from build123d import *

# Parameters (mm, degrees)
F0_W     = 65
F0_H     = 49
F0_R     = 4.5
F1_DEPTH = 1
F0_R_2   = 1.5
F3_DEPTH = 8
F4_R     = 8


with BuildPart() as f1:
    # F0 (on Top) → F1 (new body)
    with BuildSketch(Plane.XY):
        Rectangle(F0_W, F0_H)
        with Locations((-26.5, -18.5)):
            Circle(F0_R, mode=Mode.SUBTRACT)
        with Locations((26.5, -18.5)):
            Circle(F0_R, mode=Mode.SUBTRACT)
        with Locations((-26.5, 18.5)):
            Circle(F0_R, mode=Mode.SUBTRACT)
        with Locations((26.5, 18.5)):
            Circle(F0_R, mode=Mode.SUBTRACT)
    extrude(amount=F1_DEPTH)

    # F0 (on Top) → F3 (join)
    with BuildSketch(Plane.XY):
        with Locations((26.5, 18.5)):
            Circle(F0_R)
        with Locations((26.5, 18.5)):
            Circle(F0_R_2, mode=Mode.SUBTRACT)
        with Locations((-26.5, -18.5)):
            Circle(F0_R)
        with Locations((-26.5, -18.5)):
            Circle(F0_R_2, mode=Mode.SUBTRACT)
        with Locations((-26.5, 18.5)):
            Circle(F0_R)
        with Locations((-26.5, 18.5)):
            Circle(F0_R_2, mode=Mode.SUBTRACT)
        with Locations((26.5, -18.5)):
            Circle(F0_R)
        with Locations((26.5, -18.5)):
            Circle(F0_R_2, mode=Mode.SUBTRACT)
    extrude(amount=F3_DEPTH)

    # F4
    f4_edges = [f1.edges().sort_by_distance(p)[0] for p in [
        (32.5, -24.5, 0.5),
        (32.5, 24.5, 0.5),
        (-32.5, -24.5, 0.5),
        (-32.5, 24.5, 0.5),
    ]]
    fillet(f4_edges, radius=F4_R)


solid = f1.part
Model file for the job. Use its own axes, mm. A direction names the side the tool comes from. Give positions to 0.01 mm unless a question says otherwise; leave off trailing zeros. Write each loop counter-clockwise with the first axis right and the second up, starting at its lowest first coordinate (ties: lowest second). Pieces come first, ordered by that corner, then holes. Notation, with made-up numbers: (-34.75, 40.5) -> (-22.75, 40.5) arc R17 cw to (-22.75, 71.5) -> close; hole circle Ø4 at (79, 60.5). An arc over 180 degrees is marked (long way). Write item = value, one per line.
(1) Slice it at C-C, the plane y = -18.5. Give the cut face in (x, z).
Determined:
outline = (-32.25, 0) -> (-28, 0) -> (-28, 8) -> (-31, 8) -> (-31, 1) -> (-32.25, 1) -> close; (-25, 0) -> (25, 0) -> (25, 8) -> (22, 8) -> (22, 1) -> (-22, 1) -> (-22, 8) -> (-25, 8) -> close; (28, 0) -> (32.25, 0) -> (32.25, 1) -> (31, 1) -> (31, 8) -> (28, 8) -> close
(2) Probe line 1 along Y through (x, z) = (26.5, 5.25); line 2 along Z through (x, y) = (-1, -11); line 3 along X through (y, z) = (-16, 7.5). List the from-to ranges inside material, lowest first.
Determined:
line_1 = -23 to -20, -17 to -14, 14 to 17, 20 to 23
line_2 = 0 to 1
line_3 = -30.24 to -22.76, 22.76 to 30.24
(3) Flat gauge pin, fed straight in: P1, Ø2, axis at x = -2, y = 18, coming from the +Z side. Where does the tip first touch, or does it go through?
Determined:
P1 = 1
(4) Slice it at B-B, the plane x = 26.5. Give the cut face in (y, z), then the cut area to 3 significant figures.
Determined:
outline = (-24.25, 0) -> (-20, 0) -> (-20, 8) -> (-23, 8) -> (-23, 1) -> (-24.25, 1) -> close; (-17, 0) -> (17, 0) -> (17, 8) -> (14, 8) -> (14, 1) -> (-14, 1) -> (-14, 8) -> (-17, 8) -> close; (20, 0) -> (24.25, 0) -> (24.25, 1) -> (23, 1) -> (23, 8) -> (20, 8) -> close
area = 126 mm2
(5) Slice it at A-A, the plane z = 1.75. Give the cut face in (x, y).
Determined:
outline = circle Ø9 at (-26.5, -18.5); circle Ø9 at (-26.5, 18.5); circle Ø9 at (26.5, -18.5); circle Ø9 at (26.5, 18.5); hole circle Ø3 at (-26.5, -18.5); hole circle Ø3 at (-26.5, 18.5); hole circle Ø3 at (26.5, -18.5); hole circle Ø3 at (26.5, 18.5)
(6) Slice it at D-D, the plane x = -23. Give the cut face in (y, z), then the cut area to 3 significant figures.
Determined:
outline = (-24.5, 0) -> (24.5, 0) -> (24.5, 1) -> (21.33, 1) -> (21.33, 8) -> (15.67, 8) -> (15.67, 1) -> (-15.67, 1) -> (-15.67, 8) -> (-21.33, 8) -> (-21.33, 1) -> (-24.5, 1) -> close
area = 128 mm2
(7) Mould opens along Y. For faces 1 (the face through (30.094, -22.219, 0.507)), 2 (the face through (-27.09, 22.96, 4.45)), 3 (the face through (25, 20, 8)) say: released by +Y, released by -Y, zero draft, split by the parting line, or undercut.
Determined:
face_1 = released by -Y
face_2 = undercut
face_3 = zero draft
(8) Tool access for faces 4 (the face through (-27.09, -14.04, 4.45)), 5 (the face through (25.39, 19.51, 3.94)): list every direction of +Z, -Z, +X, -X, +Y, -Y with a clear straight run to the whole face (end or side of a thin tool).
Determined:
face_4 = +Z
face_5 = +Z, -Z
